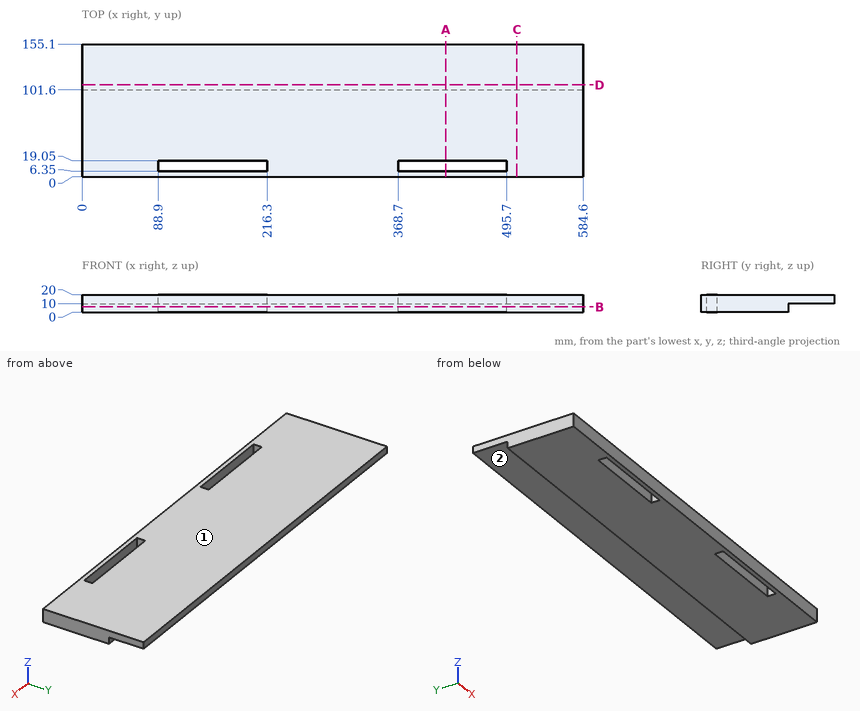
Part print with two shaded views. Sizes in mm from the minimum x, y, z corner. A direction names the side the tool comes from. Round coordinates to 2 decimals unless told otherwise and drop trailing zeros. Loops run counter-clockwise (first coordinate to the right, second up) from the corner with the lowest first, then second, coordinate; pieces in that order, holes last.
Item 1: Saw through at D-D (y = 107.5). List the corners of the cut face in (x, z).
Item 2: Pin check, flat tip, straight feed: P1, Ø6, axis at x = 199, y = 66.5, coming from the -Z side. Stop position of the tip, or through.
Item 3: Saw through at C-C (x = 507.5). List the corners of the cut face in (y, z).
Item 4: Which spindle directions (+Z, -Z, +X, -X, +Y, -Y) get a long thin tool onto all of the face, cutting with end or side? Do the marked faces 1 and 2. Say none if no direction does.
Item 5: Saw through at B-B (z = 6). List the corners of the cut face in (x, y).
Item 6: Saw through at A-A (x = 424.5). List the corners of the cut face in (y, z).
Item 7: Drill centre lines: line 1 along X through (y, z) = (8, 9.5); line 2 along Y through (x, z) = (493.5, 17.5); line 3 along Y through (x, z) = (394.5, 3.75). Where is each one in solid material? Low to high.
Worked answers:
1. outline: (0, 10) - (584.6, 10) - (584.6, 20) - (0, 20) - close
2. P1: stops at z = 0
3. outline: (0, 0) - (101.6, 0) - (101.6, 10) - (155.1, 10) - (155.1, 20) - (0, 20) - close
4. face 1: +Z, +X, -X, +Y, -Y
4. face 2: -Z, +X, -X, +Y
5. outline: (0, 0) - (584.6, 0) - (584.6, 101.6) - (0, 101.6) - close; hole (88.9, 6.35) - (216.3, 6.35) - (216.3, 19.05) - (88.9, 19.05) - close; hole (368.7, 6.35) - (495.7, 6.35) - (495.7, 19.05) - (368.7, 19.05) - close
6. outline: (0, 0) - (6.35, 0) - (6.35, 20) - (0, 20) - close; (19.05, 0) - (101.6, 0) - (101.6, 10) - (155.1, 10) - (155.1, 20) - (19.05, 20) - close
7. line 1: x = 0 to 88.9, 216.3 to 368.7, 495.7 to 584.6
7. line 2: y = 0 to 6.35, 19.05 to 155.1
7. line 3: y = 0 to 6.35, 19.05 to 101.6
